Geometry check sheet. Reference: the model listing, model coordinates, mm. A direction names the side the tool comes from. Give positions to 0.01 mm unless a question says otherwise; leave off trailing zeros. Loops run counter-clockwise (first coordinate to the right, second up) from the corner with the lowest first, then second, coordinate; pieces in that order, holes last. Notation, with made-up numbers: (11.5, -32.5) -> (64.5, -32.5) arc R16 cw to (64.5, -26.5) -> close; hole circle Ø2 at (14.5, 14.5). An arc over 180 degrees is marked (long way). One line per item, written item: value. Start each with the question number.
(1) Tool access check on faces 5 (the face through (0, -3.45, -1)), 6 (the face through (-3, -29.05, -1)), 7 (the face through (-1, -21, -0.6)). Record the directions out of +Z, -Z, +X, -X, +Y, -Y that give a thin tool (end or side, any length) a straight path to the whole face; none if there is none.
(2) Sectioned sample at B-B, the plane z = 6. State how many separate pieces and enclosed holes the cut face has, then the cut area to 3 significant figures.
(3) Sectioned sample at A-A, the plane y = -25.5. Record the cut outline in (x, z) (3 decimals).
(4) Sectioned sample at C-C, the plane y = 6.5. Record the cut outline in (x, z) (3 decimals).
(5) Scan lines: line 1 along Y through (x, z) = (0.75, 4.25); line 2 along Y through (x, z) = (-0.5, 9.75); line 3 along Y through (x, z) = (-4, 7.5). Record each from-to range of solid material in increasing order. Write a range as from..to.
(6) Gauge pin test, flat ends, axial feed: pin 1 Ø1.5 at (y, z) = (1, -1) entering from +X (3 decimals); pin 2 Ø3 at (x, y) = (-3, 5.5) entering from -Z; pin 3 Ø4 at (x, y) = (-2.5, -18.5) entering from +Z. Record the tip position at first contact, or that the pin passes through.
(7) Draft check along Y on faces 1 (the face through (-0.1, 3.25, 8.5)), 2 (the face through (0.15, -19.16, 9.75)), 3 (the face through (-8.98, -27.57, 10.43)), 4 (the face through (-7.3, 3.45, -2.7)). Enter one of: pulls with the +Y half, pulls with the -Y half, needs draft (parallel to the pull), parting line crosses it, or undercut.
Autodesk Inventor part; units mm, degrees
ref_plane "YZ Plane" through (0, 0, 0) normal (1, 0, 0) x (0, 1, 0)
ref_plane "XZ Plane" through (0, 0, 0) normal (0, 1, 0) x (-1, 0, 0)
ref_plane "XY Plane" through (0, 0, 0) normal (0, 0, 1) x (1, 0, 0)
sketch "Эскиз2" plane through (0, 0, 0) normal (0, 0, 1) x (1, 0, 0)
  line L0 (-4.5, 3.25) -> (4.5, 3.25)
  line L1 (4.5, 3.25) -> (4.5, -3.25)
  line L2 (4.5, -3.25) -> (-4.5, -3.25)
  line L3 (-4.5, -3.25) -> (-4.5, 3.25)
  line L4 (-4.5, 3.25) -> (4.5, -3.25) construction
  line L5 (4.5, 3.25) -> (-4.5, -3.25) construction
  line L6 (8.5, 9.25) -> (4.5, 9.25) construction
  line L7 (-8.5, 9.25) -> (-8.5, -5.25)
  line L8 (-8.5, -5.25) -> (4.5, -5.25)
  line L9 (8.5, -5.25) -> (8.5, 9.25) construction
  line L10 (4.5, 3.25) -> (4.5, 9.25)
  line L11 (4.5, -3.25) -> (4.5, -5.25)
  line L12 (4.5, 9.25) -> (-8.5, 9.25)
  line L13 (4.5, -5.25) -> (8.5, -5.25) construction
  point P0 (0, 0)
  dimension "d0" = 9
  dimension "d1" = 6.5
  dimension "d2" = 6
extrude "Выдавливание1" add sketch "Эскиз2" along normal blind 14 contours L3 L2 L11 L8 L7 L12 L10 L0
sketch "Эскиз4" plane through (0, 0, 0) normal (0, 0, -1) x (-1, 0, 0)
  line L0 (2.9551, -1.2625) -> (2.9551, -1.7625) construction
  line L1 (2.9551, -1.7625) -> (3.4551, -1.7625) construction
  arc A0 (3.4551, -1.7625) -> (4.305, -2.445) centre (4.405, -1.45) ccw construction
  line L2 (4.305, -2.445) -> (4.305, -3.05) construction
  line L3 (4.305, -3.05) -> (4.105, -3.25) construction
  line L4 (4.105, -3.25) -> (-4.495, -3.25) construction
  line L5 (-4.495, -3.25) -> (-4.695, -3.05) construction
  line L6 (-4.695, -3.05) -> (-4.695, -2.445) construction
  arc A1 (-4.695, -2.445) -> (-3.8451, -1.7625) centre (-4.795, -1.45) ccw construction
  line L7 (-3.8451, -1.7625) -> (-3.3451, -1.7625) construction
  line L8 (-3.3451, -1.7625) -> (-3.3451, -1.2625) construction
  line L9 (-3.3451, -1.2625) -> (-3.8127, -1.2625) construction
  arc A2 (-3.8127, -1.2625) -> (-4.695, -0.455) centre (-4.795, -1.45) ccw construction
  line L10 (-4.695, -0.455) -> (-4.695, 3.05) construction
  line L11 (-4.695, 3.05) -> (-4.495, 3.25) construction
  line L12 (-4.495, 3.25) -> (4.105, 3.25) construction
  line L13 (4.105, 3.25) -> (4.305, 3.05) construction
  line L14 (4.305, 3.05) -> (4.305, -0.455) construction
  arc A3 (4.305, -0.455) -> (3.4227, -1.2625) centre (4.405, -1.45) ccw construction
  line L15 (3.4227, -1.2625) -> (2.9551, -1.2625) construction
  line L16 (4.1878, 3.45) -> (-4.5778, 3.45) construction
  line L17 (-4.5778, 3.45) -> (-4.895, 3.1328) construction
  line L18 (-4.895, 3.1328) -> (-4.895, -0.6563) construction
  arc A4 (-3.9951, -1.4625) -> (-4.895, -0.6563) centre (-4.795, -1.45) ccw construction
  line L19 (-3.9951, -1.4625) -> (-3.5451, -1.4625) construction
  line L20 (-3.5451, -1.4625) -> (-3.5451, -1.5625) construction
  line L21 (-3.5451, -1.5625) -> (-4.0029, -1.5625) construction
  arc A5 (-4.895, -2.2437) -> (-4.0029, -1.5625) centre (-4.795, -1.45) ccw construction
  line L22 (-4.895, -2.2437) -> (-4.895, -3.1328) construction
  line L23 (-4.895, -3.1328) -> (-4.5778, -3.45) construction
  line L24 (-4.5, -3.45) -> (4.1878, -3.45)
  line L25 (4.1878, -3.45) -> (4.505, -3.1328)
  line L26 (4.505, -3.1328) -> (4.505, -2.2437)
  arc A6 (3.6129, -1.5625) -> (4.505, -2.2437) centre (4.405, -1.45) ccw
  line L27 (3.6129, -1.5625) -> (3.1551, -1.5625)
  line L28 (3.1551, -1.5625) -> (3.1551, -1.4625)
  line L29 (3.1551, -1.4625) -> (3.6051, -1.4625)
  arc A7 (4.505, -0.6563) -> (3.6051, -1.4625) centre (4.405, -1.45) ccw
  line L30 (4.505, -0.6563) -> (4.505, 3.1328)
  line L31 (4.505, 3.1328) -> (4.1878, 3.45)
  line L32 (4.1878, 3.45) -> (8.5, 3.45)
  line L33 (8.5, 9.25) -> (8.5, -5.25)
  line L34 (-4.5, -5.25) -> (-4.5, -3.25)
  line L35 (-4.5, -3.45) -> (-4.5, -29.05)
  line L36 (-4.5, -29.05) -> (10.5, -29.05)
  line L37 (10.5, -29.05) -> (10.5, 3.45)
  line L38 (10.5, 3.45) -> (8.5, 3.45)
  point P0 (0, 0)
  dimension "d10" = 0.2
  dimension "d12" = 4.3122
  dimension "d13" = 15
extrude "Выдавливание3" add sketch "Эскиз4" along normal blind 3 and the other way blind 12.4
chamfer "Фаска1" distance 2 angle 45 1 edges at (-8.5, 3.45, 6.2)
chamfer "Фаска2" distance 2 angle 45 1 edges at (-6.3439, 3.45, 0)
ref_plane "РабПлоскость1" through (0, 0, 4.7) normal (0, 0, -1) x (-1, 0, 0)
sketch "Эскиз5" plane through (0, 0, 4.7) normal (0, 0, -1) x (-1, 0, 0)
  circle A0 centre (2.8764, -21.55) radius 11 construction
  line L0 (-4.5, -29.05) -> (10.5, -29.05) construction
  circle A1 centre (2.8764, -21.55) radius 1.6
  line L1 (10.5, -29.05) -> (10.5, 3.45)
  line L2 (10.5, -29.05) -> (10.5, -9.55)
  line L3 (10.5, -9.55) -> (-4.5, -9.55)
  line L4 (-4.5, -3.45) -> (-4.5, -29.05)
  line L5 (-4.5, -9.55) -> (-4.5, -29.05)
  line L6 (-4.5, -29.05) -> (10.5, -29.05)
  point P0 (0, 0)
  dimension "d27" = 22
  dimension "d28" = 7.5
  dimension "d29" = 3.2
  dimension "d30" = 12
extrude "Выдавливание4" cut sketch "Эскиз5" along normal mid plane 7.4
extrude "Выдавливание5" cut sketch "Эскиз5" along normal mid plane 20 contours A1
sketch "Эскиз6" plane through (0, 0, -3) normal (0, 0, -1) x (-1, 0, 0)
  circle A0 centre (2.8764, -21.55) radius 1.6 construction
  circle A1 centre (2.8764, -21.55) radius 1.6
  line L0 (4.5507, -24.45) -> (1.2021, -24.45)
  line L1 (1.2021, -24.45) -> (-0.4722, -21.55)
  line L2 (-0.4722, -21.55) -> (1.2021, -18.65)
  line L3 (1.2021, -18.65) -> (4.5507, -18.65)
  line L4 (4.5507, -18.65) -> (6.2251, -21.55)
  line L5 (6.2251, -21.55) -> (4.5507, -24.45)
  line L6 (-4.5, -29.05) -> (10.5, -29.05)
  point P0 (0, 0)
  dimension "d35" = 5.8
extrude "Выдавливание6" cut sketch "Эскиз6" against normal blind 2.4
sketch "Эскиз3" plane through (-8.5, 9.25, 0) normal (0, 1, 0) x (1, 0, 0)
  line L0 (13, 0) -> (0, 0) construction
  circle A0 centre (8.695, -6.5) radius 1.75
  line L1 (13, 0) -> (13, -14)
  point P0 (8.5, 0)
  dimension "d5" = 3.5
  dimension "d9" = 4.305
extrude "Выдавливание2" cut sketch "Эскиз3" against normal blind 20
chamfer "Фаска5" distance 3 angle 45 4 edges at (-10.5, -29.05, 10.4) (-10.5, -29.05, -1) (4.5, -29.05, 10.4) (4.5, -29.05, -1)
sketch "Эскиз7" plane through (-10.5, -9.55, 8.4) normal (0, -1, 0) x (1, 0, 0)
  circle A0 centre (10.695, -1.9) radius 1.75
  circle A1 centre (10.695, -1.9) radius 3.25
  point P0 (10.5, -8.4)
  dimension "d44" = 6.5
extrude "Выдавливание7" cut sketch "Эскиз7" along normal blind 20
properties part number "ограничитель" material "Полипропилен"
Calculated:
1. face 5: -Z, +X
1. face 6: +Z, -Z, +X, -X, -Y
1. face 7: -Z
2. separate pieces: 3
2. enclosed holes: 0
2. area: 174 mm2
3. outline: (-10.5, -3) -> (4.5, -3) -> (4.5, 1) -> (-10.5, 1) -> close; (-10.5, 8.4) -> (-2.442, 8.4) arc R3.25 cw to (2.832, 8.4) -> (4.5, 8.4) -> (4.5, 12.4) -> (-10.5, 12.4) -> close
4. outline: (-8.5, 0) -> (4.5, 0) -> (4.5, 14) -> (-8.5, 14) -> close; hole circle Ø3.5 at (0.195, 6.5)
5. line 1: y = -9.55..-3.25, 3.25..9.25
5. line 2: y = -29.05..-3.25, 3.25..9.25
5. line 3: y = -9.55..-3.25, -2.14..-0.76, 3.25..9.25
6. pin 1: stops at x = -4.505
6. pin 2: stops at z = -1.35
6. pin 3: stops at z = 12.4
7. face 1: undercut
7. face 2: needs draft
7. face 3: pulls with the -Y half
7. face 4: pulls with the +Y half
